Can you work these out from the model? Positions are in its coordinate system, mm. A direction names the side the tool comes from. Coordinates: 2 decimals unless noted, no trailing zeros. Write each loop counter-clockwise with the first axis right and the second up, starting at its lowest first coordinate (ties: lowest second). Pieces come first, ordered by that corner, then holes. Notation, with made-up numbers: (52.5, 11) - (77.5, 11) arc R18 ccw to (77.5, 32) - close; hole circle Ø7 at (3.5, 57). An arc over 180 degrees is marked (long way). Use one line per item in the form item = value. Start each with the question number.
(1) Thinking about a two-plate mould opening in X: for faces 5 (the face through (-51, 21, -35)), 6 (the face through (-17.705, 20, 36)), 7 (the face through (-73.96, 1.521, -31.125)), which applies, pulls with the +X half, pulls with the -X half, needs draft (parallel to the pull), parting line crosses it, or undercut?
(2) For pin 1 Ø0.9 at (x, z) = (-54.5, -37) entering from +Y; pin 2 Ø0.9 at (y, z) = (1, -4.5) entering from -X; pin 3 Ø1.5 at (x, y) = (-13.5, 1) entering from -Z, each with a flat end and sliding along its axis, tell me the tip position at first contact or that it passes through.
(3) If we section it at D-D on z = -4.5: Please give me the cut outline in (x, y), then the cut area to 3 significant figures.
(4) If we section it at C-C on y = 5.5: Give the number of separate pieces and of enclosed holes in the cut face, then the cut area to 3 significant figures.
(5) If we section it at B-B on x = -15.5: Please give me the cut outline in (y, z).
(6) If we section it at A-A on z = 19: Please give me the cut outline in (x, y), then the cut area to 3 significant figures.
(7) If I drill on probe 1 along Z at (x, y) = (-51, 5.5); probe 2 along Z at (x, y) = (-24, 30.5); probe 3 along Y at (x, z) = (42, 13), over which ranges is the centre line in solid material (lowest first)? Write a range as from..to.
(8) On a 3-axis mill with a long thin cutter (end or side, diameter ignored), from which of +Z, -Z, +X, -X, +Y, -Y can I reach the whole of each face in a straight line? I mean faces 1 (the face through (-59, 17, -15)), 2 (the face through (51.424, 2, 0)), 3 (the face through (-49.9, 21.241, -15.285)), 4 (the face through (-12, 1, 35)). Say none if no direction works.
```python
from build123d import *

# Parameters (mm, degrees)
SKETCH_1_W           = 220
SKETCH_1_H           = 70
EXTRUDE_1_DEPTH      = 3
EXTRUDE_2_DEPTH      = 25
EXTRUDE_2_DEPTH_BACK = 25
SKETCH_6_W           = 30
SKETCH_6_H           = 37.527767497
CUT_EXTRUDE_4_DEPTH  = 221
SKETCH_7_R           = 35
CUT_EXTRUDE_5_DEPTH  = 4
SKETCH_8_W           = 3
SKETCH_8_H           = 40
EXTRUDE_3_DEPTH      = 65
SKETCH_9_R           = 1.5
CUT_EXTRUDE_6_DEPTH  = 4
FILLET_5_R           = 1
SKETCH_10_W          = 65
SKETCH_10_H          = 20
CUT_EXTRUDE_7_DEPTH  = 4
SKETCH_12_R          = 1.5
CUT_EXTRUDE_8_DEPTH  = 4


with BuildPart() as part:
    # 草图1 → 凸台-拉伸1 (new body)
    with BuildSketch(Plane(origin=(0, 0, 0), x_dir=(1, 0, 0), z_dir=(0, 1, 0))):
        with Locations((27.295373665, 0)):
            Rectangle(SKETCH_1_W, SKETCH_1_H)
    extrude(amount=EXTRUDE_1_DEPTH)

    # 草图2 → 凸台-拉伸2 (add, two sides)
    with BuildSketch(Plane.XY) as extrude_2_sk:
        Polygon((-82.704626335, 40.527767497), (-82.704626335, 3), (-17.704626335, 3), align=None)
    extrude(amount=EXTRUDE_2_DEPTH)
    extrude(extrude_2_sk.sketch, amount=-EXTRUDE_2_DEPTH_BACK)

    # 草图6 → 切除-拉伸4 (cut, through all)
    with BuildSketch(Plane.ZY.offset(82.704626335)):
        with Locations((0, 21.763883748)):
            Rectangle(SKETCH_6_W, SKETCH_6_H)
    extrude(amount=-CUT_EXTRUDE_4_DEPTH, mode=Mode.SUBTRACT)

    # 草图7 → 切除-拉伸5 (cut, through all)
    with BuildSketch(Plane(origin=(0, 3, 0), x_dir=(1, 0, 0), z_dir=(0, 1, 0))):
        with Locations((25.295373665, 51)):
            Circle(SKETCH_7_R)
        with Locations((25.295373665, -51)):
            Circle(SKETCH_7_R)
    extrude(amount=-CUT_EXTRUDE_5_DEPTH, mode=Mode.SUBTRACT)

    # 草图8 → 凸台-拉伸3 (add)
    with BuildSketch(Plane.ZY.offset(82.704626335)):
        with Locations((36.5, 20)):
            Rectangle(SKETCH_8_W, SKETCH_8_H)
        with Locations((-36.5, 20)):
            Rectangle(SKETCH_8_W, SKETCH_8_H)
    extrude(amount=-EXTRUDE_3_DEPTH)

    # 草图9 → 切除-拉伸6 (cut, through all)
    with BuildSketch(Plane(origin=(0, 3, 0), x_dir=(1, 0, 0), z_dir=(0, 1, 0))):
        with Locations((-74.766784803, 29.860059225)):
            Circle(SKETCH_9_R)
        with Locations((-54.766784803, 29.860059225)):
            Circle(SKETCH_9_R)
        with Locations((-34.766784803, 29.860059225)):
            Circle(SKETCH_9_R)
        with Locations((-34.766784803, -29.860059225)):
            Circle(SKETCH_9_R)
        with Locations((-54.766784803, -29.860059225)):
            Circle(SKETCH_9_R)
        with Locations((-74.766784803, -29.860059225)):
            Circle(SKETCH_9_R)
        with Locations((68.031562246, 22)):
            Circle(SKETCH_9_R)
        with Locations((88.031562246, 22)):
            Circle(SKETCH_9_R)
        with Locations((108.031562246, 22)):
            Circle(SKETCH_9_R)
        with Locations((108.031562246, -22)):
            Circle(SKETCH_9_R)
        with Locations((88.031562246, -22)):
            Circle(SKETCH_9_R)
        with Locations((68.031562246, -22)):
            Circle(SKETCH_9_R)
        with Locations((128.031562246, 22)):
            Circle(SKETCH_9_R)
        with Locations((128.031562246, -22)):
            Circle(SKETCH_9_R)
    extrude(amount=-CUT_EXTRUDE_6_DEPTH, mode=Mode.SUBTRACT)

    # 圆角5
    fillet_5_edges = [part.edges().sort_by_distance(p)[0] for p in [
        (-50.204626335, 21.763883749, -25),
        (-50.204626335, 21.763883749, 25),
        (-50.204626335, 21.763883749, -15),
        (-50.204626335, 21.763883749, 15),
    ]]
    fillet(fillet_5_edges, radius=FILLET_5_R)

    # 草图10 → 切除-拉伸7 (cut, through all)
    with BuildSketch(Plane(origin=(0, 3, 0), x_dir=(1, 0, 0), z_dir=(0, 1, 0))):
        with Locations((-50.204626335, 0)):
            Rectangle(SKETCH_10_W, SKETCH_10_H)
    extrude(amount=-CUT_EXTRUDE_7_DEPTH, mode=Mode.SUBTRACT)

    # 草图12 → 切除-拉伸8 (cut, through all)
    with BuildSketch(Plane(origin=(0, 3, 0), x_dir=(1, 0, 0), z_dir=(0, 1, 0))):
        with BuildLine():
            Line((51.424138498, 27.712929589), (51.424138498, 0))
            Line((51.424138498, 0), (51.424138498, -27.712929589))
            ThreePointArc((51.424138498, -27.712929589), (54.155060508, -31.198018398), (56.424138498, -35))
            Line((56.424138498, -35), (137.295373665, -35))
            Line((137.295373665, -35), (137.295373665, 35))
            Line((137.295373665, 35), (56.424138498, 35))
            ThreePointArc((56.424138498, 35), (54.155060508, 31.198018398), (51.424138498, 27.712929589))
        make_face()
        with Locations((68.031562246, -22)):
            Circle(SKETCH_12_R, mode=Mode.SUBTRACT)
        with Locations((88.031562246, -22)):
            Circle(SKETCH_12_R, mode=Mode.SUBTRACT)
        with Locations((108.031562246, -22)):
            Circle(SKETCH_12_R, mode=Mode.SUBTRACT)
        with Locations((128.031562246, -22)):
            Circle(SKETCH_12_R, mode=Mode.SUBTRACT)
        with Locations((68.031562246, 22)):
            Circle(SKETCH_12_R, mode=Mode.SUBTRACT)
        with Locations((88.031562246, 22)):
            Circle(SKETCH_12_R, mode=Mode.SUBTRACT)
        with Locations((108.031562246, 22)):
            Circle(SKETCH_12_R, mode=Mode.SUBTRACT)
        with Locations((128.031562246, 22)):
            Circle(SKETCH_12_R, mode=Mode.SUBTRACT)
    extrude(amount=-CUT_EXTRUDE_8_DEPTH, mode=Mode.SUBTRACT)


solid = part.part
```
Reported:
q1.face_5 = needs draft
q1.face_6 = pulls with the +X half
q1.face_7 = undercut
q2.pin_1 = 40
q2.pin_2 = -17.7
q2.pin_3 = -35
q3.outline = (-17.7, 0) - (51.42, 0) - (51.42, 3) - (-17.7, 3) - close
q3.area = 207 mm2
q4.separate_pieces = 4
q4.enclosed_holes = 0
q4.area = 1,600 mm2
q5.outline = (0, -35) - (3, -35) - (3, 35) - (0, 35) - close
q6.outline = (-82.7, 0) - (11.12, 0) - (11.12, 3) - (-17.7, 3) - (-82.7, 40.53) - close; (39.47, 0) - (51.42, 0) - (51.42, 3) - (39.47, 3) - close
q6.area = 1,540 mm2
q7.probe_1 = -38..-35, -25..-15, 15..25, 35..38
q7.probe_2 = -38..-35, 35..38
q7.probe_3 = 0..3
q8.face_1 = +X, -X, +Y
q8.face_2 = +Z, -Z, +X, +Y, -Y
q8.face_3 = +X, +Y
q8.face_4 = +Z, +X, +Y, -Y
